Source: CAD feature listing. Evaluate the final solid. Frame: model axes, mm. Face numbers are marked on the shaded views. A direction names the side the tool comes from. Give positions to 0.01 mm unless a question says otherwise; leave off trailing zeros. Loops run counter-clockwise (first coordinate to the right, second up) from the corner with the lowest first, then second, coordinate; pieces in that order, holes last. Notation, with made-up numbers: (9, 4.5) -> (46, 4.5) arc R24 ccw to (46, 43.5) -> close; hole circle Ø1 at (89, 19.5). An arc over 180 degrees is marked (long way). Return JSON: item names as keys, results as strings. Group by question number.
(1) Cut plane A-A on y = 0. Return loops of the section in (x, z).
(2) Pin query (flat end, axial travel): pin 1 (5 mm diameter, centred on y = 2, z = 11, fed in from -X); pin 2 (3.5 mm diameter, centred on x = -10.5, y = 1.5, fed in from +Z); pin 3 (2 mm diameter, centred on x = 2.5, z = 4.5, fed in from +Y). Return the tip coordinate at first contact, or that it passes through.
(3) Cut plane C-C on x = -11.5. Return loops of the section in (y, z).
(4) Access query for the marked faces 1 and 2. Directions: +Z, -Z, +X, -X, +Y, -Y. A direction counts if a zero-diameter tool reaches every point of the face in a straight line with its end or side. Return the directions, or none.
(5) Cut plane B-B on x = 5. Return loops of the section in (y, z), then the cut area to 3 significant figures.
(6) Ray query, line 1 (Z direction, x = -5, y = 3.5); line 2 (Y direction, x = -2.25, z = 6); line 3 (X direction, y = -0.25, z = 7.25). Return the intervals inside material, ascending. Write a range as from..to.
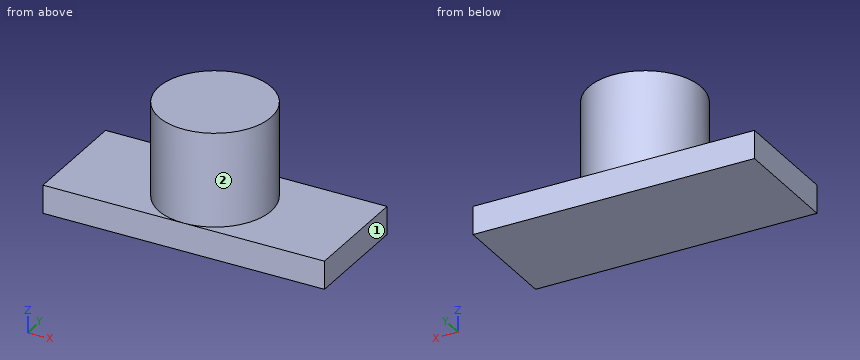
Autodesk Inventor part; units mm, degrees
ref_plane "YZ Plane" through (0, 0, 0) normal (1, 0, 0) x (0, 1, 0)
ref_plane "XZ Plane" through (0, 0, 0) normal (0, 1, 0) x (-1, 0, 0)
ref_plane "XY Plane" through (0, 0, 0) normal (0, 0, 1) x (1, 0, 0)
sketch "Sketch1" plane through (0, 0, 0) normal (0, 0, 1) x (1, 0, 0)
  line L0 (-15, 6) -> (15, 6)
  line L1 (15, 6) -> (15, -6)
  line L2 (15, -6) -> (-15, -6)
  line L3 (-15, -6) -> (-15, 6)
  line L4 (-15, 6) -> (15, -6) construction
  line L5 (15, 6) -> (-15, -6) construction
  point P0 (0, 0)
  dimension "d0" = 30
  dimension "d1" = 12
extrude "Extrusion1" add sketch "Sketch1" along normal blind 3
sketch "Sketch2" plane through (0, 0, 3) normal (0, 0, 1) x (1, 0, 0)
  circle A0 centre (0, 0) radius 6
  dimension "d4" = 12
extrude "Extrusion2" add sketch "Sketch2" along normal blind 10
thread "Thread2"
properties part number "BOTTOM STOPPER" material "Steel, Alloy"
Answers:
{
 "1": {"outline": "(-15, 0) -> (15, 0) -> (15, 3) -> (6, 3) -> (6, 13) -> (-6, 13) -> (-6, 3) -> (-15, 3) -> close"},
 "2": {"pin 1": "x = -6", "pin 2": "z = 3", "pin 3": "y = 5.81"},
 "3": {"outline": "(-6, 0) -> (6, 0) -> (6, 3) -> (-6, 3) -> close"},
 "4": {"face 1": "+Z, -Z, +X, +Y, -Y", "face 2": "+Z"},
 "5": {"outline": "(-6, 0) -> (6, 0) -> (6, 3) -> (3.32, 3) -> (3.32, 13) -> (-3.32, 13) -> (-3.32, 3) -> (-6, 3) -> close", "area": "102 mm²"},
 "6": {"line 1": "0..3", "line 2": "-5.56..5.56", "line 3": "-5.99..5.99"}
}
